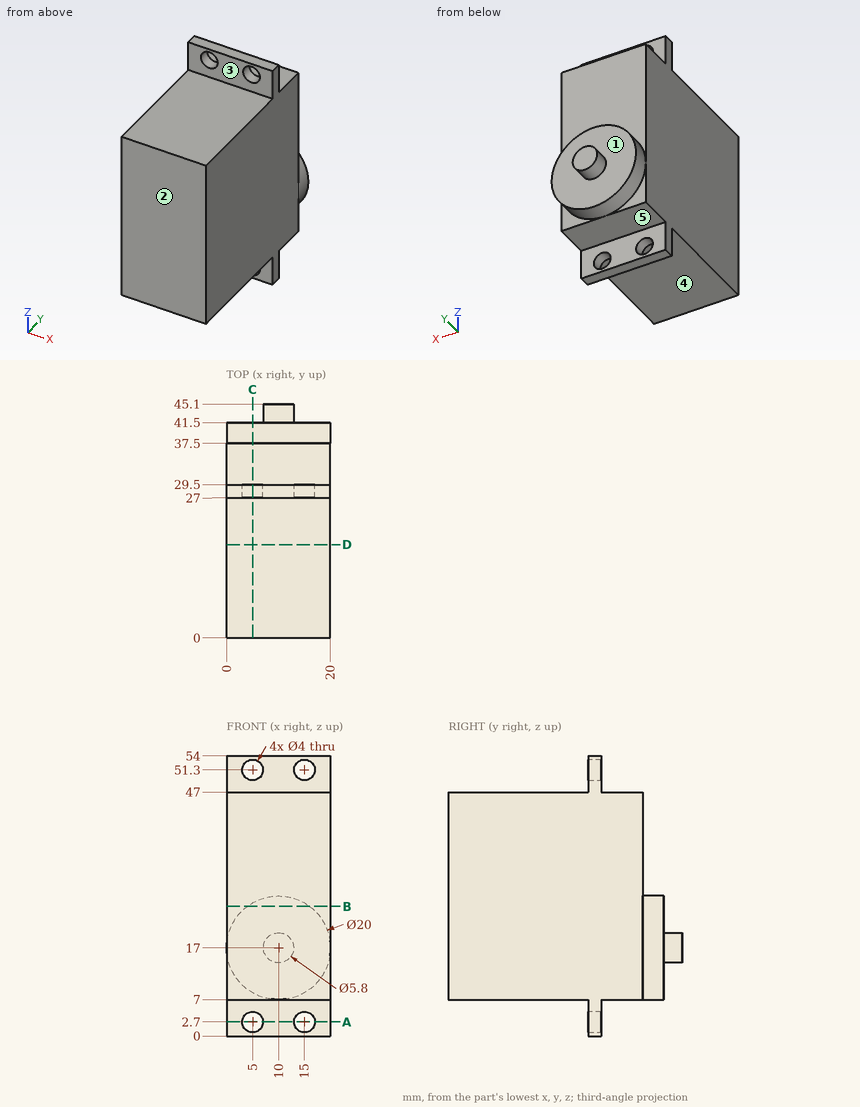
Print and shaded views of the part. All mm, measured from the part's lowest x, y and z. A direction names the side the tool comes from. Round coordinates to 2 decimals unless told otherwise and drop trailing zeros. Write each loop counter-clockwise with the first axis right and the second up, starting at its lowest first coordinate (ties: lowest second). Pieces come first, ordered by that corner, then holes. Notation, with made-up numbers: (61.25, 63) - (85.25, 63) arc R36 cw to (85.25, 100) - close; hole circle Ø5 at (62, 42.5). An arc over 180 degrees is marked (long way). One line per question, with ' | ' between items.
1. Drill centre lines: line 1 along X through (y, z) = (28.05, 51.3); line 2 along X through (y, z) = (28, 2); line 3 along Z through (x, y) = (1, 18). Where is each one in solid material? Low to high. Write a range as from..to.
Results are:
line 1: 0..3, 7..13, 17..20 | line 2: 0..3.13, 6.87..13.13, 16.87..20 | line 3: 7..47
2. Drop flat-ended pins along their axis: pin 1 Ø6 at (x, z) = (9.5, 29.5) entering from +Y; pin 2 Ø8 at (x, y) = (4, 18) entering from +Z; pin 3 Ø1.5 at (x, y) = (10.5, 18.5) entering from -Z; pin 4 Ø3 at (x, z) = (5, 51.3) entering from +Y. Give the stop position or say it passes through.
Results are:
pin 1: y = 41.5 | pin 2: z = 47 | pin 3: z = 7 | pin 4: through
3. Band-saw the part on A-A, the plane z = 2.7. Write the cut outline in (x, y), and give its area (3 significant figures).
Results are:
outline: (0, 27) - (3, 27) - (3, 29.5) - (0, 29.5) - close; (7, 27) - (13, 27) - (13, 29.5) - (7, 29.5) - close; (17, 27) - (20, 27) - (20, 29.5) - (17, 29.5) - close | area: 30.0 mm^2
4. Band-saw the part on B-B, the plane z = 25. Write the cut outline in (x, y).
Results are:
outline: (0, 0) - (20, 0) - (20, 37.5) - (16, 37.5) - (16, 41.5) - (4, 41.5) - (4, 37.5) - (0, 37.5) - close
5. Tool access for the marked faces 1, 2, 3, 4 and 5: list every direction of +Z, -Z, +X, -X, +Y, -Y with a clear straight run to the whole face (end or side of a thin tool).
Results are:
face 1: +Y | face 2: +Z, -Z, +X, -X, -Y | face 3: +Z, +X, -X, -Y | face 4: -Z, +X, -X, -Y | face 5: -Z, +X, -X, +Y
6. Band-saw the part on D-D, the plane y = 18. Write the cut outline in (x, z).
Results are:
outline: (0, 7) - (20, 7) - (20, 47) - (0, 47) - close
7. Band-saw the part on C-C, the plane x = 5. Write the cut outline in (y, z), and give its area (3 significant figures).
Results are:
outline: (0, 7) - (27, 7) - (27, 4.7) - (29.5, 4.7) - (29.5, 7) - (37.5, 7) - (37.5, 8.34) - (41.5, 8.34) - (41.5, 25.66) - (37.5, 25.66) - (37.5, 47) - (29.5, 47) - (29.5, 49.3) - (27, 49.3) - (27, 47) - (0, 47) - close; (27, 0) - (29.5, 0) - (29.5, 0.7) - (27, 0.7) - close; (27, 53.3) - (29.5, 53.3) - (29.5, 54) - (27, 54) - close | area: 1,580 mm^2
